from build123d import *

# Parameters (mm, degrees)
SKETCH1_R                       = 5.7
BOSS_EXTRUDE1_DEPTH             = 8
TAP_DRILL_FOR_M3X0_5_TAP1_D     = 2.5
TAP_DRILL_FOR_M3X0_5_TAP1_DEPTH = 5
TAP_DRILL_FOR_M3X0_5_TAP1_TIP   = 0.751075774
TAP_DRILL_FOR_M3X0_5_TAP2_D     = 2.5
TAP_DRILL_FOR_M3X0_5_TAP2_DEPTH = 5
TAP_DRILL_FOR_M3X0_5_TAP2_TIP   = 0.751075774
TAP_DRILL_FOR_M3X0_5_TAP3_D     = 2.5
TAP_DRILL_FOR_M3X0_5_TAP3_DEPTH = 5
TAP_DRILL_FOR_M3X0_5_TAP3_TIP   = 0.751075774
SKETCH8_R                       = 8
CUT_EXTRUDE1_DEPTH              = 2.1


with BuildPart() as part:
    # Sketch1 → Boss-Extrude1 (new body)
    with BuildSketch(Plane.XY):
        with BuildLine():
            Line((0, 0), (39, 0))
            Line((39, 0), (39, 8))
            Line((39, 8), (33, 8))
            ThreePointArc((33, 8), (30, 11), (33, 14))
            Line((33, 14), (39, 14))
            Line((39, 14), (39, 22))
            Line((39, 22), (0, 22))
            Line((0, 22), (0, 14))
            Line((0, 14), (6, 14))
            ThreePointArc((6, 14), (9, 11), (6, 8))
            Line((6, 8), (0, 8))
            Line((0, 8), (0, 0))
        make_face()
        with Locations((19.5, 11)):
            Circle(SKETCH1_R, mode=Mode.SUBTRACT)
    extrude(amount=BOSS_EXTRUDE1_DEPTH)

    # Tap Drill for M3x0.5 Tap1
    with Locations(Plane(origin=(39, 0, 0), x_dir=(0, 0, -1), z_dir=(1, 0, 0))):
        with Locations((-4, 18), (-4, 4)):
            Hole(TAP_DRILL_FOR_M3X0_5_TAP1_D / 2, depth=TAP_DRILL_FOR_M3X0_5_TAP1_DEPTH)
            with Locations((0, 0, -(TAP_DRILL_FOR_M3X0_5_TAP1_DEPTH + TAP_DRILL_FOR_M3X0_5_TAP1_TIP / 2))):  # 118° drill point
                Cone(0, TAP_DRILL_FOR_M3X0_5_TAP1_D / 2, TAP_DRILL_FOR_M3X0_5_TAP1_TIP, mode=Mode.SUBTRACT)

    # Tap Drill for M3x0.5 Tap2
    with Locations(Plane.ZY):
        with Locations((4, 4), (4, 18)):
            Hole(TAP_DRILL_FOR_M3X0_5_TAP2_D / 2, depth=TAP_DRILL_FOR_M3X0_5_TAP2_DEPTH)
            with Locations((0, 0, -(TAP_DRILL_FOR_M3X0_5_TAP2_DEPTH + TAP_DRILL_FOR_M3X0_5_TAP2_TIP / 2))):  # 118° drill point
                Cone(0, TAP_DRILL_FOR_M3X0_5_TAP2_D / 2, TAP_DRILL_FOR_M3X0_5_TAP2_TIP, mode=Mode.SUBTRACT)

    # Tap Drill for M3x0.5 Tap3
    with Locations(Plane(origin=(0, 22, 0), x_dir=(1, 0, 0), z_dir=(0, 1, 0))):
        with Locations((31, -4), (8, -4)):
            Hole(TAP_DRILL_FOR_M3X0_5_TAP3_D / 2, depth=TAP_DRILL_FOR_M3X0_5_TAP3_DEPTH)
            with Locations((0, 0, -(TAP_DRILL_FOR_M3X0_5_TAP3_DEPTH + TAP_DRILL_FOR_M3X0_5_TAP3_TIP / 2))):  # 118° drill point
                Cone(0, TAP_DRILL_FOR_M3X0_5_TAP3_D / 2, TAP_DRILL_FOR_M3X0_5_TAP3_TIP, mode=Mode.SUBTRACT)

    # Sketch8 → Cut-Extrude1 (cut)
    with BuildSketch(Plane(origin=(0, 0, 0), x_dir=(-1, 0, 0), z_dir=(0, 0, -1))):
        with Locations((-19.5, 11)):
            Circle(SKETCH8_R)
    extrude(amount=-CUT_EXTRUDE1_DEPTH, mode=Mode.SUBTRACT)


solid = part.part
Geometry check sheet. Reference: the model listing, model coordinates, mm. A direction names the side the tool comes from. Round coordinates to 2 decimals unless told otherwise and drop trailing zeros. Order: outer loops, then holes, each group sorted by start corner. A loop starts at its lowest first (then second) coordinate and runs counter-clockwise, first axis right, second up. Notation, with made-up numbers: M -24,86.25 L 16,86.25 A17 cw 16,113.25 Z; hole C -32.75,-27.5 d9. An arc over 180 degrees is marked long. Answer in a Markdown table with one row per item. Add a question column.
Item 1: Draft check along X on faces 6 (the face through (36, 8, 4)), 7 (the face through (15.299, 14.852, 5.009)), 8 (the face through (39, 3, 3)). Enter one of: released by +X, released by -X, zero draft, split by the parting line, or undercut.
Item 2: Set-up check for faces 1 (the face through (3, 14, 4)), 2 (the face through (25.849, 6.132, 1.035)), 3 (the face through (36, 14, 4)), 4 (the face through (29.845, 19.465, 4.479)), 5 (the face through (36.47, 16.78, 3.73)): record each of +Z, -Z, +X, -X, +Y, -Y from which the full face is reachable in a straight line by a thin tool's end or side.
Item 3: Sectioned sample at C-C, the plane x = 19.5. Enter the section's corners in (y, z).
Item 4: Material ranges on L1, parallel to Y at x = 35.4, z = 4; L2, parallel to Y at x = 19.5, z = 6.75; L3, parallel to Z at x = 31, y = 20.55, recorded low to high. Write a range as [from, to].
Item 5: Depth check by flat-ended pin: pin 1 Ø2 at (y, z) = (4, 4) entering from +X; pin 2 Ø9.5 at (x, y) = (19.5, 11) entering from -Z. Enter the tip coordinate at first touch or a pass-through.
Item 6: Sectioned sample at B-B, the plane y = 11. Enter the section's corners in (x, z).
Item 7: Sectioned sample at A-A, the plane z = 1.5. Enter the section's corners in (x, y).
Item 8: Sectioned sample at D-D, the plane z = 7. Enter the section's corners in (x, y), plus the area to 3 significant figures.
Filled in:
| question | item | result |
|---|---|---|
| 1 | face 6 | zero draft |
| 1 | face 7 | undercut |
| 1 | face 8 | released by +X |
| 2 | face 1 | +Z, -Z, -X |
| 2 | face 2 | -Z |
| 2 | face 3 | +Z, -Z, +X |
| 2 | face 4 | +Y |
| 2 | face 5 | +X |
| 3 | outline | M 0,0 L 3,0 L 3,2.1 L 5.3,2.1 L 5.3,8 L 0,8 Z; M 16.7,2.1 L 19,2.1 L 19,0 L 22,0 L 22,8 L 16.7,8 Z |
| 4 | L1 | y = [0, 2.75], [5.25, 8], [14, 16.75], [19.25, 22] |
| 4 | L2 | y = [0, 5.3], [16.7, 22] |
| 4 | L3 | z = [0, 2.75], [5.25, 8] |
| 5 | pin 1 | stops at x = 33.85 |
| 5 | pin 2 | passes through |
| 6 | outline | M 9,0 L 11.5,0 L 11.5,2.1 L 13.8,2.1 L 13.8,8 L 9,8 Z; M 25.2,2.1 L 27.5,2.1 L 27.5,0 L 30,0 L 30,8 L 25.2,8 Z |
| 7 | outline | M 0,0 L 39,0 L 39,8 L 33,8 A3 cw 33,14 L 39,14 L 39,22 L 0,22 L 0,14 L 6,14 A3 cw 6,8 L 0,8 Z; hole C 19.5,11 d16 |
| 8 | outline | M 0,0 L 39,0 L 39,8 L 33,8 A3 cw 33,14 L 39,14 L 39,22 L 0,22 L 0,14 L 6,14 A3 cw 6,8 L 0,8 Z; hole C 19.5,11 d11.4 |
| 8 | area | 656 mm² |
